The drawing under review shows one solid part. Ordinate dimensions are in mm from its lowest x, y, z. Coordinates: 2 decimals unless noted, no trailing zeros. Write each loop counter-clockwise with the first axis right and the second up, starting at its lowest first coordinate (ties: lowest second). Pieces come first, ordered by that corner, then holes. Notation, with made-up numbers: (-13, 51.25) -> (-7, 51.25) arc R19 cw to (-7, 73.25) -> close; hole circle Ø2 at (21, 6). An arc over 180 degrees is marked (long way). One line per item, written item: value. Start each with the question number.
1) Add section C-C (y = 72). State the section outline as (x, z) points.
2) For probe 1 along Y at (x, z) = (30, 5); probe 2 along Y at (x, z) = (102.5, 3.25); probe 3 along X at (y, z) = (75, 6), list the stretches that pass through material, from the lowest coordinate up. Write a range as from..to.
3) Add section D-D (x = 98). State the section outline as (y, z) points, and give its area (3 significant figures).
4) Add section A-A (x = 65). State the section outline as (y, z) points, and give its area (3 significant figures).
5) For pin 1 Ø1.9 at (x, z) = (23.5, 3) entering from +Y; pin 2 Ø3 at (y, z) = (2, 2) entering from -X, all flat-tipped, find the tip position at first contact; note any pin that passes through.
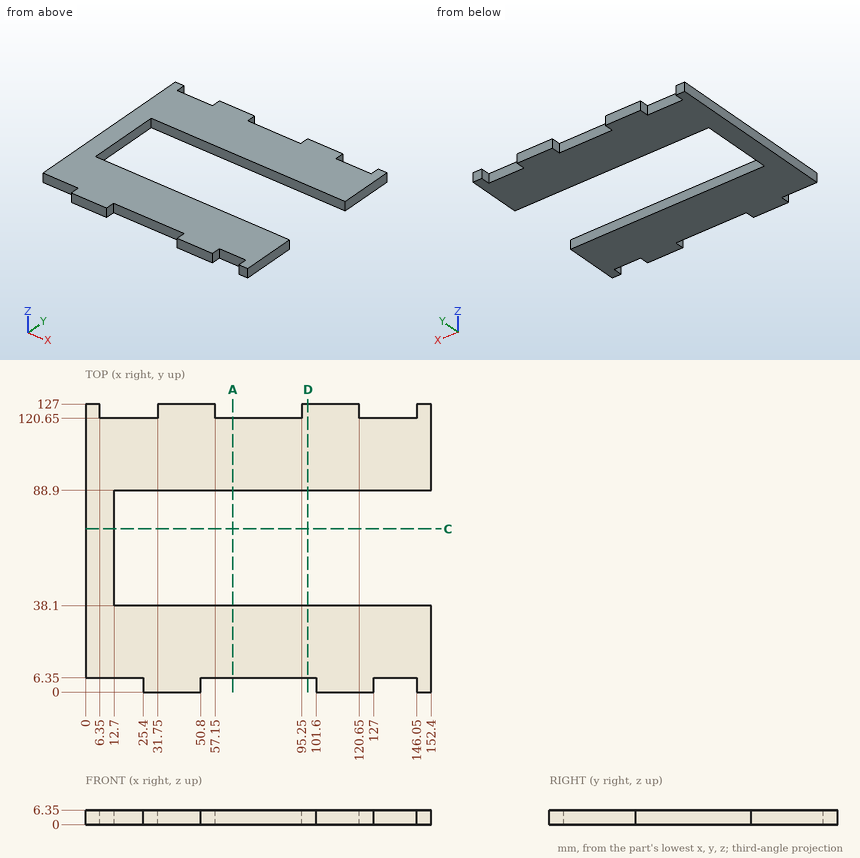
Numbers:
1. outline: (0, 0) -> (12.7, 0) -> (12.7, 6.35) -> (0, 6.35) -> close
2. probe 1: 0..38.1, 88.9..120.65
2. probe 2: 0..38.1, 88.9..127
2. probe 3: 0..12.7
3. outline: (6.35, 0) -> (38.1, 0) -> (38.1, 6.35) -> (6.35, 6.35) -> close; (88.9, 0) -> (127, 0) -> (127, 6.35) -> (88.9, 6.35) -> close
3. area: 444 mm²
4. outline: (6.35, 0) -> (38.1, 0) -> (38.1, 6.35) -> (6.35, 6.35) -> close; (88.9, 0) -> (120.65, 0) -> (120.65, 6.35) -> (88.9, 6.35) -> close
4. area: 403 mm²
5. pin 1: y = 120.65
5. pin 2: x = 25.4
